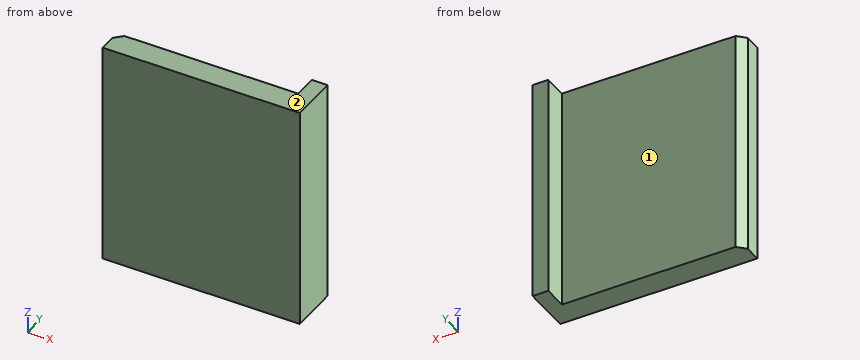
from build123d import *

# Parameters (mm, degrees)
SKETCH1_W           = 25
SKETCH1_H           = 28.5
BOSS_EXTRUDE1_DEPTH = 3.3
SKETCH2_W           = 2
SKETCH2_H           = 28.5
BOSS_EXTRUDE2_DEPTH = 3
CHAMFER1_SIZE       = 1
SKETCH3_R           = 21.891628128
CUT_EXTRUDE1_DEPTH  = 0.2


with BuildPart() as part:
    # Sketch1 → Boss-Extrude1 (new body)
    with BuildSketch(Plane(origin=(0, 0, 0), x_dir=(1, 0, 0), z_dir=(0, 1, 0))):
        with Locations((-3.305606618, -1.571691176)):
            Rectangle(SKETCH1_W, SKETCH1_H)
    extrude(amount=BOSS_EXTRUDE1_DEPTH)

    # Sketch2 → Boss-Extrude2 (add)
    with BuildSketch(Plane(origin=(0, 3.3, 0), x_dir=(1, 0, 0), z_dir=(0, 1, 0))):
        with Locations((8.194393382, -1.571691176)):
            Rectangle(SKETCH2_W, SKETCH2_H)
    extrude(amount=BOSS_EXTRUDE2_DEPTH)

    # Chamfer1
    chamfer1_edges = [part.edges().sort_by_distance(p)[0] for p in [
        (-15.805606618, 3.3, 1.571691176),
    ]]
    chamfer(chamfer1_edges, length=CHAMFER1_SIZE)

    # Sketch3 → Cut-Extrude1 (cut)
    with BuildSketch(Plane.XZ):
        with Locations((-2.847820653, 0)):
            Circle(SKETCH3_R)
    extrude(amount=-CUT_EXTRUDE1_DEPTH, mode=Mode.SUBTRACT)


solid = part.part
Source: CAD feature listing. Evaluate the final solid. Frame: model axes, mm. Face numbers are marked on the shaded views. A direction names the side the tool comes from. Round coordinates to 2 decimals unless told otherwise and drop trailing zeros. Loops run counter-clockwise (first coordinate to the right, second up) from the corner with the lowest first, then second, coordinate; pieces in that order, holes last. Notation, with made-up numbers: (39, -2.75) -> (58, -2.75) arc R26 ccw to (58, 27.25) -> close; hole circle Ø3 at (18, -21.5). An arc over 180 degrees is marked (long way). Answer as a JSON object with one key per item and string values. Group by question number.
Q1. Section query B-B (y = 3.75). Output: boundary loops of the cut face in (x, z), plus the area to 3 significant figures.
Q2. Ray query, line 1 (Y direction, x = -8.5, z = -5.75); line 2 (X direction, y = 5, z = 6.75); line 3 (X direction, y = 3.25, z = -0.25). Return the intervals inside material, ascending. Write a range as from..to.
Q3. Section query C-C (x = -7.25). Output: boundary loops of the cut face in (y, z).
Q4. Access query for the marked faces 1 and 2. Directions: +Z, -Z, +X, -X, +Y, -Y. A direction counts if a zero-diameter tool reaches every point of the face in a straight line with its end or side. Return the directions, or none.
Q5. Section query A-A (z = -5.5). Output: boundary loops of the cut face in (x, y), plus the area to 3 significant figures.
Q6. Contact query for flat-ended pins moving along their axis: P1, Ø2, axis at x = 1.5, z = -7.5, coming from the +Y side; P2, Ø2.5, axis at y = 4.5, z = 0, coming from the -X side. Output: stop coordinate, or through.
Completed:
{
 "1": {"outline": "(7.19, -12.68) -> (9.19, -12.68) -> (9.19, 15.82) -> (7.19, 15.82) -> close", "area": "57.0 mm²"},
 "2": {"line 1": "0.2..3.3", "line 2": "7.19..9.19", "line 3": "-14.86..9.19"},
 "3": {"outline": "(0.2, -12.68) -> (3.3, -12.68) -> (3.3, 15.82) -> (0.2, 15.82) -> close"},
 "4": {"face 1": "+Z, -Z, -X, +Y", "face 2": "+Z, +X, -X, +Y, -Y"},
 "5": {"outline": "(-15.81, 0.2) -> (9.19, 0.2) -> (9.19, 6.3) -> (7.19, 6.3) -> (7.19, 3.3) -> (-14.81, 3.3) -> (-15.81, 2.3) -> close", "area": "83.0 mm²"},
 "6": {"P1": "y = 3.3", "P2": "x = -14.86"}
}
